```python
from build123d import *

# Parameters (mm, degrees)
F1_DEPTH = 6
F2_R     = 0.5
F3_DEPTH = 10
F4_R     = 0.5
F5_DEPTH = 10
F6_R     = 0.5
F7_DEPTH = 10


with BuildPart() as f1:
    # F0 (on Top) → F1 (new body)
    with BuildSketch(Plane.XY):
        Polygon((-3, 1.7320508076), (-3, -1.7320508076), (0, -3.4641016151), (3, -1.7320508076), (3, 1.7320508076), (0, 3.4641016151), align=None)
        Polygon((0, -2.8867513459), (-2.5, -1.443375673), (-2.5, 1.443375673), (0, 2.8867513459), (2.5, 1.443375673), (2.5, -1.443375673), align=None, mode=Mode.SUBTRACT)
    extrude(amount=F1_DEPTH)

    # F2 (on face) → F3 (cut)
    with BuildSketch(Plane.YZ.offset(3)):
        with Locations((0, 2.8977813589)):
            Circle(F2_R)
    extrude(amount=-F3_DEPTH, mode=Mode.SUBTRACT)

    # F4 (on face) → F5 (cut)
    with BuildSketch(Plane(origin=(1.5, 2.5980762114, 0), x_dir=(-0.8660254038, 0.5, 0), z_dir=(0.5, 0.8660254038, 0))):
        with Locations((0, 2.9807699823)):
            Circle(F4_R)
    extrude(amount=-F5_DEPTH, mode=Mode.SUBTRACT)

    # F6 (on face) → F7 (cut)
    with BuildSketch(Plane(origin=(-1.5, 2.5980762114, 0), x_dir=(-0.8660254038, -0.5, 0), z_dir=(-0.5, 0.8660254038, 0))):
        with Locations((0.2181102464, 2.9651848599)):
            Circle(F6_R)
    extrude(amount=-F7_DEPTH, mode=Mode.SUBTRACT)


solid = f1.part
```
Could you check a few things on this model? Use its own coordinates, in mm. A direction names the side the tool comes from. Round coordinates to 2 decimals unless told otherwise and drop trailing zeros. Write each loop counter-clockwise with the first axis right and the second up, starting at its lowest first coordinate (ties: lowest second). Pieces come first, ordered by that corner, then holes.
(1) Suppose I cut it at B-B on z = 5.4. Write out the boundary of the cut face in (x, y).
Findings below:
outline: (-3, -1.73) - (0, -3.46) - (3, -1.73) - (3, 1.73) - (0, 3.46) - (-3, 1.73) - close; hole (-2.5, -1.44) - (0, -2.89) - (2.5, -1.44) - (2.5, 1.44) - (0, 2.89) - (-2.5, 1.44) - close
(2) Which directions (+Z, -Z, +X, -X, +Y, -Y) give clear straight access to the entire face, cutting with the end or side of a thin tool? Please do faces 4 (the face through (-0.677, -2.496, 2.958)), 5 (the face through (1.5, -2.6, 2.3)).
Findings below:
face 4: +Z, -Z
face 5: +Z, -Z, +X, -Y
(3) Thinking about a two-plate mould opening in Z: for faces 1 (the face through (2, -2, 0)), 2 (the face through (-1.5, 2.6, 2.3)), 3 (the face through (1.471, 2.33, 2.493)), which applies, +Z half, -Z half, draft (parallel to the pull), parting line (faces both ways), or undercut?
Findings below:
face 1: -Z half
face 2: draft
face 3: undercut
(4) Suppose I cut it at D-D on y = 0.75. Write out the boundary of the cut face in (x, z).
Findings below:
outline: (-3, 0) - (-2.5, 0) - (-2.5, 6) - (-3, 6) - close; (2.5, 0) - (3, 0) - (3, 6) - (2.5, 6) - close
(5) Suppose I cut it at A-A on y = 0. Write out the boundary of the cut face in (x, z).
Findings below:
outline: (-3, 0) - (-2.5, 0) - (-2.5, 2.4) - (-3, 2.4) - close; (-3, 3.4) - (-2.5, 3.4) - (-2.5, 6) - (-3, 6) - close; (2.5, 0) - (3, 0) - (3, 2.4) - (2.5, 2.4) - close; (2.5, 3.4) - (3, 3.4) - (3, 6) - (2.5, 6) - close
(6) Suppose I cut it at C-C on x = -0.5. Write out the boundary of the cut face in (y, z).
Findings below:
outline: (-3.18, 0) - (-2.6, 0) - (-2.6, 6) - (-3.18, 6) - close; (2.6, 0) - (3.18, 0) - (3.18, 6) - (2.6, 6) - close
(7) If I drill on probe 1 along Z at (x, y) = (2.8, 0); probe 2 along X at (y, z) = (0.75, 1.4); probe 3 along X at (y, z) = (-2, 1.1), over which ranges is the centre line in solid material (lowest first)?
Findings below:
probe 1: z = 0 to 2.4, 3.4 to 6
probe 2: x = -3 to -2.5, 2.5 to 3
probe 3: x = -2.54 to -1.54, 1.54 to 2.54
